```python
from build123d import *

# Parameters (mm, degrees)
EXTRUDE_THIN1_DEPTH = 99
CHAMFER1_SIZE       = 0.5
FILLET1_R           = 2
SKETCH2_W           = 1.5
SKETCH2_H           = 0.8
SKETCH2_W_2         = 0.8
SKETCH2_H_2         = 1.5
CUT_EXTRUDE1_DEPTH  = 100.814828558


# Read off the part's stored shape, not the designer's step: Mirror1
with BuildPart() as part:
    # Sketch1 → Extrude-Thin1 (new body)
    with BuildSketch(Plane(origin=(0, 0, 0), x_dir=(0, 1, 0), z_dir=(0, 0, 1))):
        Polygon((9, 1), (1, 1), (1, 9), (-1, 9), (-1, -1), (9, -1), align=None)
    extrude(amount=EXTRUDE_THIN1_DEPTH)

    # Chamfer1
    chamfer1_edges = [part.edges().sort_by_distance(p)[0] for p in [
        (1, -1, 49.5),
    ]]
    chamfer(chamfer1_edges, length=CHAMFER1_SIZE)

    # Fillet1
    fillet1_edges = [part.edges().sort_by_distance(p)[0] for p in [
        (-1, 1, 49.5),
    ]]
    fillet(fillet1_edges, radius=FILLET1_R)

    # Sketch2 → Cut-Extrude1 (cut, through all)
    with BuildSketch(Plane.XY.offset(99)):
        with Locations((-8.25, -0.6)):
            Rectangle(SKETCH2_W, SKETCH2_H)
        with Locations((0.6, 8.25)):
            Rectangle(SKETCH2_W_2, SKETCH2_H_2)
    extrude(amount=-CUT_EXTRUDE1_DEPTH, mode=Mode.SUBTRACT)

    # Sketch5 → CSK for M3 Flat Head Machine Screw1 (revolve, cut)
    with BuildSketch(Plane(origin=(1, 4, 3.4), x_dir=(0, 0, -1), z_dir=(0, 1, 0))):
        Polygon((0, 0), (0, 10), (1.7, 10), (1.7, 1.45), (3.15, 0), align=None)
    revolve(axis=Axis((7.35, 4, 3.4), (-1, 0, 0)), mode=Mode.SUBTRACT)

    # Sketch5 at point 2 (carried to point 2, square into its face) → CSK for M3 Flat Head Machine Screw1 at 2 (revolve, cut)
    with BuildSketch(Plane(origin=(-4, -1, 8.3), x_dir=(0, 0, -1), z_dir=(1, 0, 0))):
        Polygon((0, 0), (0, 10), (1.7, 10), (1.7, 1.45), (3.15, 0), align=None)
    revolve(axis=Axis((-4, -7.35, 8.3), (0, 1, 0)), mode=Mode.SUBTRACT)

    # Mirror1 outline → Mirror1 (revolve, cut)
    with BuildSketch(Plane(origin=(-4, 0, 90.7), x_dir=(1, 0, 0), z_dir=(0, 0, 1))):
        Polygon((1.7, 0.45), (1.7, 1.126574026), (0, 1.126574026), (0, -1), (3.15, -1), align=None)
    revolve(axis=Axis((-4, 0, 90.7), (0, 1, 0)), mode=Mode.SUBTRACT)

    # Mirror1 2 outline → Mirror1 2 (revolve, cut)
    with BuildSketch(Plane(origin=(0, 4, 95.6), x_dir=(0, 1, 0), z_dir=(0, 0, -1))):
        Polygon((0, -1.126574026), (1.7, -1.126574026), (1.7, -0.45), (3.15, 1), (0, 1), align=None)
    revolve(axis=Axis((0, 4, 95.6), (1, 0, 0)), mode=Mode.SUBTRACT)


solid = part.part
```
Geometry: final body of the model. Coordinates: model frame, mm. A direction names the side the tool comes from. Give positions to 0.01 mm unless a question says otherwise; leave off trailing zeros. Loops run counter-clockwise (first coordinate to the right, second up) from the corner with the lowest first, then second, coordinate; pieces in that order, holes last. Notation, with made-up numbers: (-9.5, 2.25) -> (48.5, 2.25) arc R22 cw to (48.5, 28.25) -> close; hole circle Ø11 at (81, 56). An arc over 180 degrees is marked (long way). Return JSON: item names as keys, results as strings.
Item 1: Section A-A, the plane y = 4. Output: boundary loops of the cut face in (x, z).
Filled in:
{"outline": "(-1, 0) -> (1, 0) -> (1, 0.25) -> (-0.45, 1.7) -> (-1, 1.7) -> close; (-1, 5.1) -> (-0.45, 5.1) -> (1, 6.55) -> (1, 92.45) -> (-0.45, 93.9) -> (-1, 93.9) -> close; (-1, 97.3) -> (-0.45, 97.3) -> (1, 98.75) -> (1, 99) -> (-1, 99) -> close"}
Item 2: Mould query, pull axis X, two halves, no side actions, for faces 1 (the flat face through (1, 3, 49)), 2 (the flat face through (-1, 6, 49)), 3 (the flat face through (-1, 2, 99)), 4 (the cylindrical face through (-2.38, 0.72, 90.19)). Classes: released by +X, released by -X, zero draft, split by the parting line, or undercut.
Filled in:
{"face 1": "released by +X", "face 2": "released by -X", "face 3": "zero draft", "face 4": "undercut"}
Item 3: Pin query (flat end, axial travel): P1, Ø1.8, axis at x = -7, z = 29.5, coming from the +Y side; P2, Ø5.5, axis at y = 4, z = 95.6, coming from the +X side; P3, Ø0.8, axis at x = -8, z = 43, coming from the -Y side. Return the tip coordinate at first contact, or that it passes through.
Filled in:
{"P1": "y = 1", "P2": "x = 0.6", "P3": "y = -0.2"}
Item 4: Section C-C, the plane z = 3.4. Output: boundary loops of the cut face in (x, y), plus the area to 3 significant figures.
Filled in:
{"outline": "(-9, -0.2) -> (-7.5, -0.2) -> (-7.5, -1) -> (0.5, -1) -> (1, -0.5) -> (1, 0.85) -> (-0.45, 2.3) -> (-1.13, 2.3) arc R2 cw to (-3, 1) -> (-9, 1) -> close; (-1, 5.7) -> (-0.45, 5.7) -> (1, 7.15) -> (1, 7.5) -> (0.2, 7.5) -> (0.2, 9) -> (-1, 9) -> close", "area": "25.4 mm^2"}
Item 5: Section B-B, the plane x = -4. Output: boundary loops of the cut face in (y, z), plus the area to 3 significant figures.
Filled in:
{"outline": "(-1, 0) -> (1, 0) -> (1, 6.6) -> (0.45, 6.6) -> (-1, 5.15) -> close; (-1, 11.45) -> (0.45, 10) -> (1, 10) -> (1, 89) -> (0.45, 89) -> (-1, 87.55) -> close; (-1, 93.85) -> (0.45, 92.4) -> (1, 92.4) -> (1, 99) -> (-1, 99) -> close", "area": "180 mm^2"}
Item 6: Line query: line 1 (Z direction, x = -4, y = 0.95); line 2 (X direction, y = 0.7, z = 8.3); line 3 (Z direction, x = -0.5, y = 4.75). Output: solid intervals per line, ascending.
Filled in:
{"line 1": "0 to 6.6, 10 to 89, 92.4 to 99", "line 2": "-9 to -5.7, -2.3 to 1", "line 3": "0 to 1.87, 4.93 to 94.07, 97.13 to 99"}
Item 7: Access query for faces 5 (the flat face through (-6, 1, 49)), 6 (the cylindrical face through (-0.71, 2.3, 95.67)). Directions: +Z, -Z, +X, -X, +Y, -Y. A direction counts if a zero-diameter tool reaches every point of the face in a straight line with its end or side. Return the directions, or none.
Filled in:
{"face 5": "+Z, -Z, -X, +Y", "face 6": "+X, -X"}
Item 8: Section D-D, the plane z = 49.5. Output: boundary loops of the cut face in (x, y).
Filled in:
{"outline": "(-9, -0.2) -> (-7.5, -0.2) -> (-7.5, -1) -> (0.5, -1) -> (1, -0.5) -> (1, 7.5) -> (0.2, 7.5) -> (0.2, 9) -> (-1, 9) -> (-1, 3) arc R2 cw to (-3, 1) -> (-9, 1) -> close"}
